Drawing for the job (mm, zero at the part's lowest x, y, z). A direction names the side the tool comes from. Coordinates: 2 decimals unless noted, no trailing zeros. Order: outer loops, then holes, each group sorted by start corner. A loop starts at its lowest first (then second) coordinate and runs counter-clockwise, first axis right, second up.
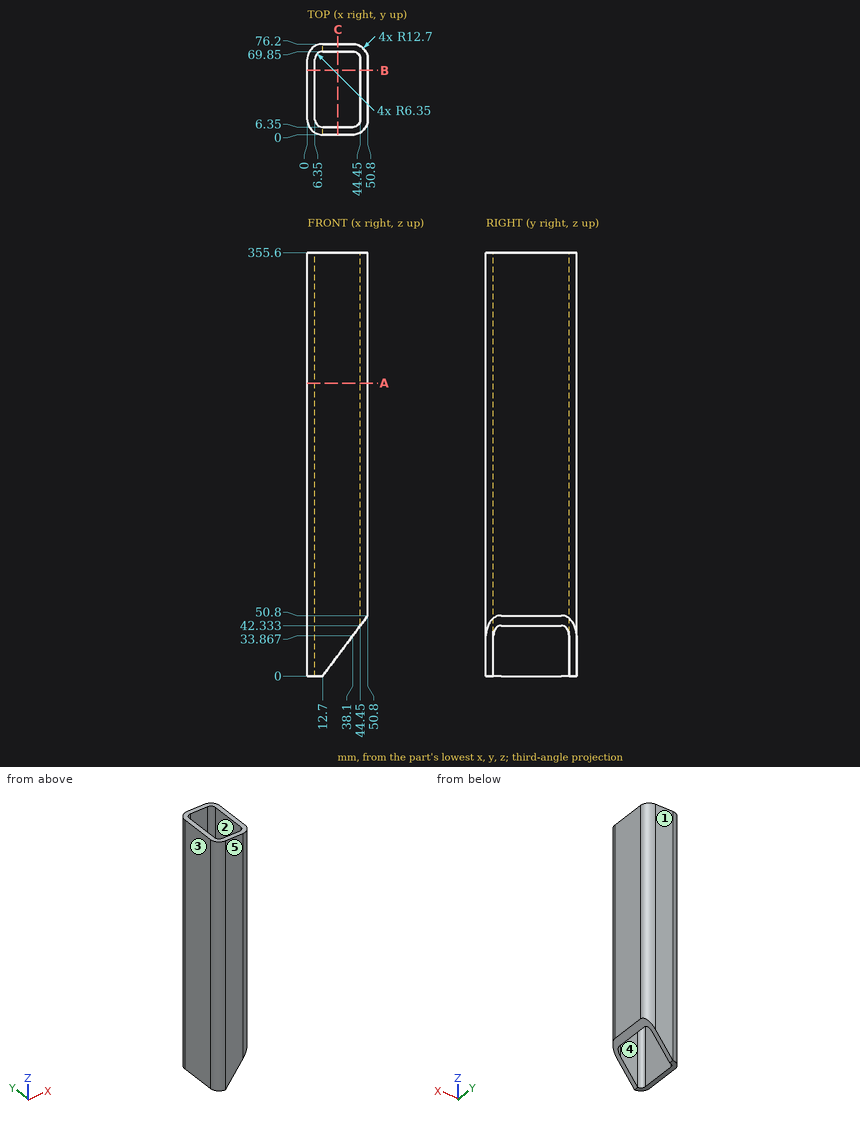
(1) Slice it at C-C, the plane x = 25.5. Give the cut face in (y, z).
(2) Drop a flat-ended pin along its axis: pin 1 (1.5 mm diameter, centred on x = 45.5, z = 175, fed in from -Y). Give the stop position or say it passes through.
(3) Slice it at A-A, the plane z = 246. Give the cut face in (x, y).
(4) Slice it at B-B, the plane y = 54. Give the cut face in (x, z), then the cut area to 3 significant figures.
(5) Pull direction Y, two halves, no side cores. Call the marked faces 3, 4 and 5: +Y half, -Y half, draft (parallel to the pull), parting line (faces both ways), or undercut.
(6) Probe line 1 (X direction, y = 13, z = 330); line 2 (Y direction, x = 28.5, z = 193.5); line 3 (Y direction, x = 41.5, z = 306.5) (1 decimal). List the from-to ranges inside material, lowest first.
(7) Tool access for the marked faces 1 and 2: list every direction of +Z, -Z, +X, -X, +Y, -Y with a clear straight run to the whole face (end or side of a thin tool).
Here are the results:
1. outline: (0, 17.07) - (6.35, 17.07) - (6.35, 355.6) - (0, 355.6) - close; (69.85, 17.07) - (76.2, 17.07) - (76.2, 355.6) - (69.85, 355.6) - close
2. pin 1: stops at y = 1.88
3. outline: (0, 12.7) arc R12.7 ccw to (12.7, 0) - (38.1, 0) arc R12.7 ccw to (50.8, 12.7) - (50.8, 63.5) arc R12.7 ccw to (38.1, 76.2) - (12.7, 76.2) arc R12.7 ccw to (0, 63.5) - close; hole (6.35, 12.7) arc R6.35 ccw to (12.7, 6.35) - (38.1, 6.35) arc R6.35 ccw to (44.45, 12.7) - (44.45, 63.5) arc R6.35 ccw to (38.1, 69.85) - (12.7, 69.85) arc R6.35 ccw to (6.35, 63.5) - close
4. outline: (0, 0) - (6.35, 0) - (6.35, 355.6) - (0, 355.6) - close; (44.45, 42.33) - (50.8, 50.8) - (50.8, 355.6) - (44.45, 355.6) - close
4. area: 4,220 mm2
5. face 3: draft
5. face 4: undercut
5. face 5: -Y half
6. line 1: x = 0 to 6.35, 44.45 to 50.8
6. line 2: y = 0 to 6.35, 69.85 to 76.2
6. line 3: y = 0.5 to 7.3, 68.9 to 75.7
7. face 1: +Z, -Z, +X, -X, +Y
7. face 2: +Z, -Z
